```python
from build123d import *

# Parameters (mm, degrees)
SKETCH1_W                      = 40
SKETCH1_H                      = 40
SKETCH1_W_2                    = 36
SKETCH1_H_2                    = 36
BOSS_EXTRUDE1_DEPTH            = 350
M4_CLEARANCE_HOLE1_D           = 4.3
M4_CLEARANCE_HOLE1_DEPTH       = 2
M4_CLEARANCE_HOLE1_TIP         = 1.291850331
SKETCH5_W                      = 35
SKETCH5_H                      = 35
CUT_EXTRUDE1_DEPTH             = 2
F_4_4_4_4_DIAMETER_HOLE1_D     = 4.4
M3_CLEARANCE_HOLE1_D           = 3.4
M3_CLEARANCE_HOLE1_DEPTH       = 20
M3_CLEARANCE_HOLE1_TIP         = 1.021463052
CUT_EXTRUDE2_REACH             = 356.542
CUT_EXTRUDE2_DIRECTION_2_DEPTH = 355.541958025


with BuildPart() as part:
    # Sketch1 → Boss-Extrude1 (new body)
    with BuildSketch(Plane(origin=(0, 0, 0), x_dir=(0, 0, -1), z_dir=(1, 0, 0))):
        with Locations((20, 20)):
            Rectangle(SKETCH1_W, SKETCH1_H)
        with Locations((20, 20)):
            Rectangle(SKETCH1_W_2, SKETCH1_H_2, mode=Mode.SUBTRACT)
    extrude(amount=BOSS_EXTRUDE1_DEPTH)

    # M4 Clearance Hole1
    with Locations(Plane.XY):
        with Locations((279.706395966, 30.606601718), (300.919599401, 30.606601718), (300.919599401, 9.393398282), (279.706395966, 9.393398282)):
            Hole(M4_CLEARANCE_HOLE1_D / 2, depth=M4_CLEARANCE_HOLE1_DEPTH)
            with Locations((0, 0, -(M4_CLEARANCE_HOLE1_DEPTH + M4_CLEARANCE_HOLE1_TIP / 2))):  # 118° drill point
                Cone(0, M4_CLEARANCE_HOLE1_D / 2, M4_CLEARANCE_HOLE1_TIP, mode=Mode.SUBTRACT)

    # Sketch5 → Cut-Extrude1 (cut)
    with BuildSketch(Plane(origin=(0, 0, -40), x_dir=(-1, 0, 0), z_dir=(0, 0, -1))):
        with Locations((-290.312997684, 20)):
            Rectangle(SKETCH5_W, SKETCH5_H)
    extrude(amount=-CUT_EXTRUDE1_DEPTH, mode=Mode.SUBTRACT)

    # Ø4.4 (4.4) Diameter Hole1 (through all)
    with Locations(Plane(origin=(0, 0, -2), x_dir=(-1, 0, 0), z_dir=(0, 0, -1))):
        with Locations((-290.312997684, 20)):
            Hole(F_4_4_4_4_DIAMETER_HOLE1_D / 2)

    # M3 Clearance Hole1
    with Locations(Plane.XY.offset(-38)):
        with Locations((6.75, 9), (20.25, 31), (13.5, 31), (6.75, 31), (20.25, 9), (13.5, 9)):
            Hole(M3_CLEARANCE_HOLE1_D / 2, depth=M3_CLEARANCE_HOLE1_DEPTH)
            with Locations((0, 0, -(M3_CLEARANCE_HOLE1_DEPTH + M3_CLEARANCE_HOLE1_TIP / 2))):  # 118° drill point
                Cone(0, M3_CLEARANCE_HOLE1_D / 2, M3_CLEARANCE_HOLE1_TIP, mode=Mode.SUBTRACT)

    # Sketch11 → Cut-Extrude2 (cut, up to next)
    with BuildSketch(Plane.XY, mode=Mode.PRIVATE) as cut_extrude2_sk1:
        with BuildLine():
            Line((6, 35), (21, 35))
            ThreePointArc((21, 35), (23.121320344, 34.121320344), (24, 32))
            Line((24, 32), (24, 8))
            ThreePointArc((24, 8), (23.121320344, 5.878679656), (21, 5))
            Line((21, 5), (6, 5))
            ThreePointArc((6, 5), (3.878679656, 5.878679656), (3, 8))
            Line((3, 8), (3, 32))
            ThreePointArc((3, 32), (3.878679656, 34.121320344), (6, 35))
        make_face()
    cut_extrude2_tool1 = extrude(cut_extrude2_sk1.sketch, amount=-CUT_EXTRUDE2_REACH, mode=Mode.PRIVATE) & part.part
    add(cut_extrude2_tool1.solids().sort_by_distance((13.5, 20, 0))[0], mode=Mode.SUBTRACT)

    # Sketch11 → Cut-Extrude2 direction 2 (cut)
    with BuildSketch(Plane.XY):
        with BuildLine():
            Line((6, 35), (21, 35))
            ThreePointArc((21, 35), (23.121320344, 34.121320344), (24, 32))
            Line((24, 32), (24, 8))
            ThreePointArc((24, 8), (23.121320344, 5.878679656), (21, 5))
            Line((21, 5), (6, 5))
            ThreePointArc((6, 5), (3.878679656, 5.878679656), (3, 8))
            Line((3, 8), (3, 32))
            ThreePointArc((3, 32), (3.878679656, 34.121320344), (6, 35))
        make_face()
    extrude(amount=CUT_EXTRUDE2_DIRECTION_2_DEPTH, mode=Mode.SUBTRACT)


solid = part.part
```
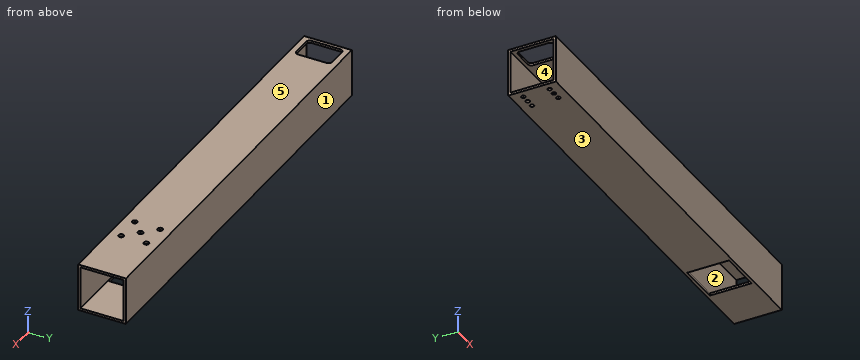
Input: part model. Units: mm. Frame: model coordinates. Face numbers are marked on the shaded views. A direction names the side the tool comes from. Give positions to 0.01 mm unless a question says otherwise; leave off trailing zeros. Order: outer loops, then holes, each group sorted by start corner. A loop starts at its lowest first (then second) coordinate and runs counter-clockwise, first axis right, second up. Notation, with made-up numbers: M -7,63.25 L 22,63.25 A13 ccw 22,76.25 Z; hole C 65.5,47 d9. An arc over 180 degrees is marked long. Return JSON: item names as keys, results as strings.
Item 1: First-contact query: P1, Ø4, axis at x = 6.75, y = 31, coming from the +Z side. Flat tip, straight axial feed; report the tip coordinate or a pass-through.
Solutions:
{"P1": "z = -38"}
Item 2: Ray query, probe 1 along Z at (x, y) = (46, 3); probe 2 along Y at (x, z) = (205, -26); probe 3 along Y at (x, z) = (6.75, -38.7). Return the intervals inside material, ascending.
Solutions:
{"probe 1": "-40 to -38, -2 to 0", "probe 2": "0 to 2, 38 to 40", "probe 3": "0 to 7.3, 10.7 to 29.3, 32.7 to 40"}
Item 3: Cut plane A-A (z = -10). Return loops of the section in (x, y).
Solutions:
{"outline": "M 0,0 L 350,0 L 350,2 L 0,2 Z; M 0,38 L 350,38 L 350,40 L 0,40 Z"}
Item 4: Pull-direction query (Y, two-part tool) for the marked faces 1, 2 and 3; classes: +Y half, -Y half, draft (parallel to the pull), parting line (faces both ways), or undercut.
Solutions:
{"face 1": "+Y half", "face 2": "undercut", "face 3": "draft"}
Item 5: Access query for the marked faces 4 and 5. Directions: +Z, -Z, +X, -X, +Y, -Y. A direction counts if a zero-diameter tool reaches every point of the face in a straight line with its end or side. Return the directions, or none.
Solutions:
{"face 4": "+X, -X", "face 5": "+Z, +X, -X, +Y, -Y"}
Item 6: Cut plane B-B (x = 118). Return loops of the section in (y, z), then the cut area to 3 significant figures.
Solutions:
{"outline": "M 0,-40 L 40,-40 L 40,0 L 0,0 Z; hole M 2,-38 L 38,-38 L 38,-2 L 2,-2 Z", "area": "304 mm^2"}
